```python
from build123d import *

# Parameters (mm, degrees)
SKETCH1_R           = 5
BOSS_EXTRUDE1_DEPTH = 5
BOSS_EXTRUDE2_DEPTH = 30
FILLET1_R           = 5
SKETCH7_R           = 2.6
CUT_EXTRUDE1_DEPTH  = 30


with BuildPart() as part:
    # Sketch1 → Boss-Extrude1 (new body)
    with BuildSketch(Plane.XY):
        with BuildLine():
            Line((-9.070221734, 4.313108884), (-25, -30))
            Line((-25, -30), (-25, -40))
            Line((-25, -40), (25, -40.363582182))
            Line((25, -40.363582182), (25, -30))
            Line((25, -30), (9.070221734, 4.313108884))
            ThreePointArc((9.070221734, 4.313108884), (0, 10.102280261), (-9.070221734, 4.313108884))
        make_face()
        Circle(SKETCH1_R, mode=Mode.SUBTRACT)
    extrude(amount=BOSS_EXTRUDE1_DEPTH)

    # Sketch6 → Boss-Extrude2 (add)
    with BuildSketch(Plane.XY.offset(5)):
        Polygon((-25, -35), (-25, -40), (25, -40.363582182), (25, -35.363582182), align=None)
    extrude(amount=BOSS_EXTRUDE2_DEPTH)

    # Fillet1
    fillet1_edges = [part.edges().sort_by_distance(p)[0] for p in [
        (0, -35.181791091, 5),
    ]]
    fillet(fillet1_edges, radius=FILLET1_R)

    # Sketch7 → Cut-Extrude1 (cut)
    with BuildSketch(Plane(origin=(-0.255815921, -35.179930889, 0), x_dir=(0.9999735626477819, -0.0072714514027518145, 0), z_dir=(0.007271451402751815, 0.999973562647782, 0))):
        with Locations(Location((-12.244838267, -23, 0), (0, 0, 180))):
            Circle(SKETCH7_R)
    cut_extrude1 = extrude(amount=-CUT_EXTRUDE1_DEPTH, mode=Mode.SUBTRACT)

    # Mirror2: Cut-Extrude1 across plane
    add(cut_extrude1.mirror(Plane(origin=(0, 0, 0), x_dir=(0, 0, 1), z_dir=(1, 0, 0))), mode=Mode.SUBTRACT)


solid = part.part
```
Can you work these out from the model? Positions are in its coordinate system, mm. A direction names the side the tool comes from. Coordinates: 2 decimals unless noted, no trailing zeros. Loops run counter-clockwise (first coordinate to the right, second up) from the corner with the lowest first, then second, coordinate; pieces in that order, holes last. Notation, with made-up numbers: (40, 18.5) -> (53, 18.5) arc R38 ccw to (53, 56.5) -> close; hole circle Ø6 at (82.25, -16.5). An arc over 180 degrees is marked (long way). Put each result on its own line as item: value. Start each with the question number.
Q1. For faces 4 (the face through (25, -38, 13)), 5 (the face through (-0.36, -33.68, 6.43)), which set-ups out of +Z, -Z, +X, -X, +Y, -Y let a thin tool reach every point of the face, with its end or its side?
Q2. I'm going to push flat-ended pins straight in: P1, Ø10, axis at x = -3, z = 12, coming from the +Y side; P2, Ø5, axis at x = -8, z = 13.5, coming from the +Y side; P3, Ø12, axis at x = 12, y = -19.5, coming from the +Z side. Where does each tip first touch, or does it pass through?
Q3. I want a section at B-B (z = 11). Write out the boundary of the cut face in (x, y).
Q4. If I drill on line 1 (Z direction, x = -13.5, y = -23.5); line 2 (Y direction, x = 0, z = 3); line 3 (Y direction, x = 6, z = 22.5), over which ranges is the centre line in solid material (lowest first)? Write a range as [from, to].
Q5. I want a section at A-A (y = 0). Write out the boundary of the cut face in (x, z), plus the area to 3 significant figures.
Q6. I want a section at C-C (y = -28). Write out the boundary of the cut face in (x, z).
Q7. Thinking about a two-plate mould opening in X: for faces 1 (the face through (-16.92, -12.6, 2.47)), 2 (the face through (-1.08, -4.88, 2.46)), 3 (the face through (0, -14, 5)), which applies, pulls with the +X half, pulls with the -X half, needs draft (parallel to the pull), parting line crosses it, or undercut?
Taken from the geometry:
1. face 4: +Z, -Z, +X, +Y, -Y
1. face 5: +Z, +X, +Y
2. P1: stops at y = -34.16
2. P2: stops at y = -35.11
2. P3: stops at z = 5
3. outline: (-25, -40) -> (25, -40.36) -> (25, -35.36) -> (-25, -35) -> close
4. line 1: z = [0, 5]
4. line 2: y = [-40.18, -5], [5, 10.1]
4. line 3: y = [-40.23, -35.23]
5. outline: (-11.07, 0) -> (-5, 0) -> (-5, 5) -> (-11.07, 5) -> close; (5, 0) -> (11.07, 0) -> (11.07, 5) -> (5, 5) -> close
5. area: 60.7 mm2
6. outline: (-24.07, 0) -> (24.07, 0) -> (24.07, 5) -> (-24.07, 5) -> close
7. face 1: pulls with the -X half
7. face 2: undercut
7. face 3: needs draft
